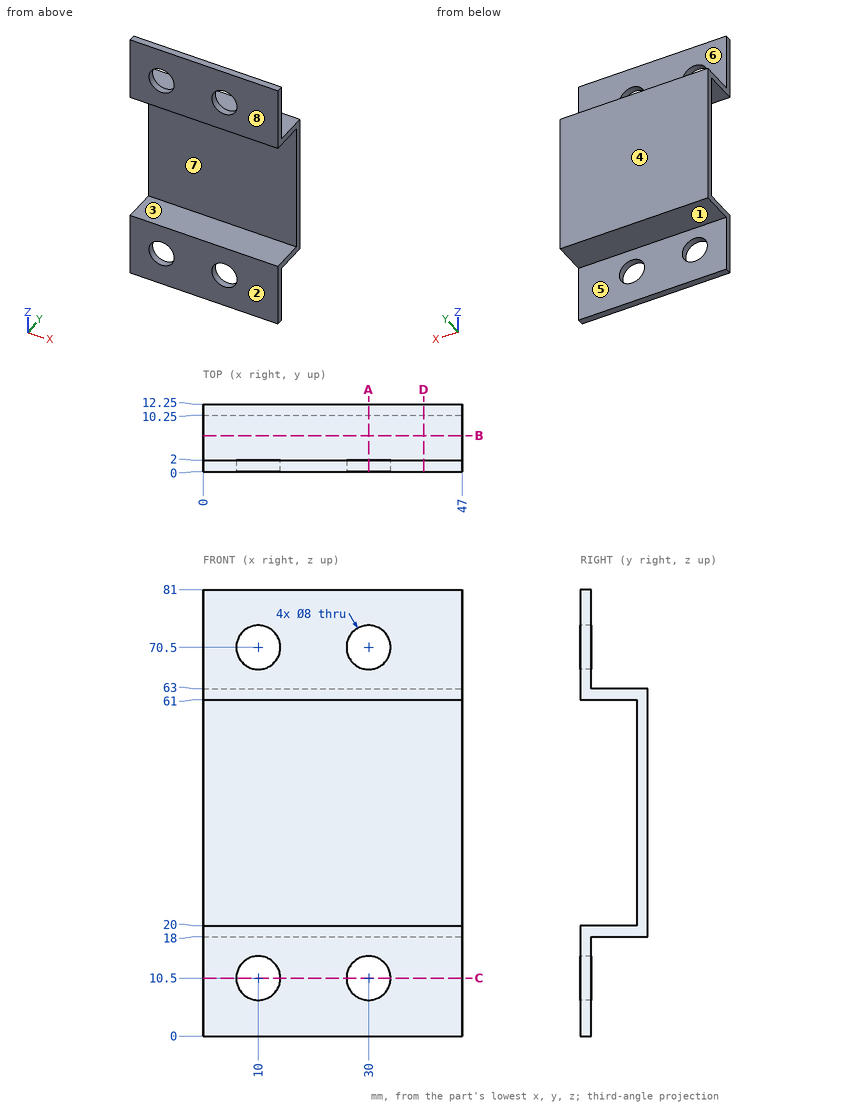
Design review of the part shown in the three views and the two pictorial views. Dimensions are in mm from the part's minimum x, y and z. A direction names the side the tool comes from. Round coordinates to 2 decimals unless told otherwise and drop trailing zeros. Loops run counter-clockwise (first coordinate to the right, second up) from the corner with the lowest first, then second, coordinate; pieces in that order, holes last. Notation, with made-up numbers: (40, -22) - (94, -22) arc R21 cw to (94, 15) - close; hole circle Ø10 at (37.25, -22.5). An arc over 180 degrees is marked (long way). One line per item, written item: value. Start each with the question number.
Item 1: For the marked faces 4, 5, 6, 7 and 8, list the 3-axis set-ups (+Z, -Z, +X, -X, +Y, -Y) from which the entire face can be reached by the end or side of a thin tool; tool diameter is ignored.
Item 2: The part is to be moulded in two halves that separate along Z. For the marked faces 1, 2 and 3, say which applies: +Z half, -Z half, draft (parallel to the pull), parting line (faces both ways), or undercut.
Item 3: Clearance check with flat-ended pins moving along their axes: pin 1 Ø14.5 at (x, z) = (33, 67.5) entering from +Y; pin 2 Ø13 at (x, z) = (10, 10.5) entering from +Y; pin 3 Ø10 at (x, z) = (27.5, 34.5) entering from -Y. State where each tip first meets the part, or that it passes through.
Item 4: Take a section at B-B (y = 6.5). Give the boundary of the cut face in (x, z).
Item 5: For L1, parallel to Z at x = 30, y = 1.55; L2, parallel to Z at x = 31.5, y = 6.75; L3, parallel to Z at x = 40, y = 0.5, list the stretches that pass through material, from the lowest coordinate up.
Item 6: Take a section at A-A (x = 30). Give the boundary of the cut face in (y, z).
Item 7: Take a section at D-D (x = 40). Give the boundary of the cut face in (y, z).
Item 8: Take a section at C-C (z = 10.5). Give the boundary of the cut face in (x, y).
Answer below:
1. face 4: +Z, -Z, +X, -X, +Y
1. face 5: -Z, +X, -X, +Y
1. face 6: +Z, +X, -X, +Y
1. face 7: +X, -X, -Y
1. face 8: +Z, -Z, +X, -X, -Y
2. face 1: -Z half
2. face 2: draft
2. face 3: undercut
3. pin 1: stops at y = 12.25
3. pin 2: stops at y = 2
3. pin 3: stops at y = 10.25
4. outline: (0, 18) - (47, 18) - (47, 20) - (0, 20) - close; (0, 61) - (47, 61) - (47, 63) - (0, 63) - close
5. L1: z = 0 to 6.5, 14.5 to 20, 61 to 66.5, 74.5 to 81
5. L2: z = 18 to 20, 61 to 63
5. L3: z = 0 to 20, 61 to 81
6. outline: (0, 0) - (2, 0) - (2, 6.5) - (0, 6.5) - close; (0, 14.5) - (2, 14.5) - (2, 18) - (12.25, 18) - (12.25, 63) - (2, 63) - (2, 66.5) - (0, 66.5) - (0, 61) - (10.25, 61) - (10.25, 20) - (0, 20) - close; (0, 74.5) - (2, 74.5) - (2, 81) - (0, 81) - close
7. outline: (0, 0) - (2, 0) - (2, 18) - (12.25, 18) - (12.25, 63) - (2, 63) - (2, 81) - (0, 81) - (0, 61) - (10.25, 61) - (10.25, 20) - (0, 20) - close
8. outline: (0, 0) - (6, 0) - (6, 2) - (0, 2) - close; (14, 0) - (26, 0) - (26, 2) - (14, 2) - close; (34, 0) - (47, 0) - (47, 2) - (34, 2) - close
